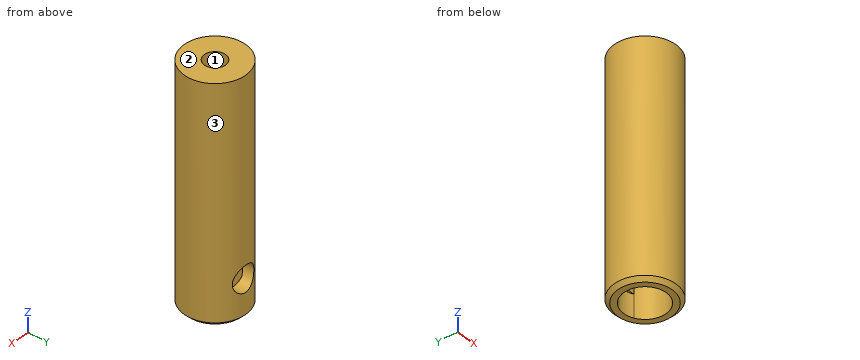
```python
from build123d import *

# Parameters (mm, degrees)
ESQUISSE1_R             = 4.075
BOSS_EXTRU_1_DEPTH      = 30.6
ENL_V_MAT_EXTRU_1_DEPTH = 14
ESQUISSE3_R             = 2.8
ENL_V_MAT_EXTRU_2_DEPTH = 3
CHANFREIN1_SIZE         = 0.5
ESQUISSE5_R             = 1.4
ENL_V_MAT_EXTRU_4_DEPTH = 10
D_GAGEMENT_M31_D        = 3.4
D_GAGEMENT_M31_DEPTH    = 4
D_GAGEMENT_M31_TIP      = 1.021463052


with BuildPart() as part:
    # Esquisse1 → Boss.-Extru.1 (new body)
    with BuildSketch(Plane.XY):
        Circle(ESQUISSE1_R)
    extrude(amount=BOSS_EXTRU_1_DEPTH)

    # Esquisse2 → Enlèv. mat.-Extru.1 (cut)
    with BuildSketch(Plane(origin=(0, 0, 0), x_dir=(-1, 0, 0), z_dir=(0, 0, -1))):
        with BuildLine():
            Line((-1.260952021, 2.5), (1.260952021, 2.5))
            ThreePointArc((1.260952021, 2.5), (0, -2.8), (-1.260952021, 2.5))
        make_face()
    extrude(amount=-ENL_V_MAT_EXTRU_1_DEPTH, mode=Mode.SUBTRACT)

    # Esquisse3 → Enlèv. mat.-Extru.2 (cut)
    with BuildSketch(Plane(origin=(0, 0, 0), x_dir=(-1, 0, 0), z_dir=(0, 0, -1))):
        Circle(ESQUISSE3_R)
    extrude(amount=-ENL_V_MAT_EXTRU_2_DEPTH, mode=Mode.SUBTRACT)

    # Chanfrein1
    chanfrein1_edges = [part.edges().sort_by_distance(p)[0] for p in [
        (-4.075, 0, 0),
    ]]
    chamfer(chanfrein1_edges, length=CHANFREIN1_SIZE)

    # Esquisse5 → Enlèv. mat.-Extru.4 (cut)
    with BuildSketch(Plane.XY.offset(30.6)):
        Circle(ESQUISSE5_R)
    extrude(amount=-ENL_V_MAT_EXTRU_4_DEPTH, mode=Mode.SUBTRACT)

    # Dégagement M31
    with Locations(Plane(origin=(0, 4.075, 0), x_dir=(1, 0, 0), z_dir=(0, 1, 0))):
        with Locations((0, -5)):
            Hole(D_GAGEMENT_M31_D / 2, depth=D_GAGEMENT_M31_DEPTH)
            with Locations((0, 0, -(D_GAGEMENT_M31_DEPTH + D_GAGEMENT_M31_TIP / 2))):  # 118° drill point
                Cone(0, D_GAGEMENT_M31_D / 2, D_GAGEMENT_M31_TIP, mode=Mode.SUBTRACT)


solid = part.part
```
Check sheet for the modelled part. Datum: model origin and axes. Units: mm. Face numbers are marked on the shaded views. Round coordinates to 2 decimals unless told otherwise and drop trailing zeros. Loops run counter-clockwise (first coordinate to the right, second up) from the corner with the lowest first, then second, coordinate; pieces in that order, holes last. Notation, with made-up numbers: (37, 28.5) - (89, 28.5) arc R30 cw to (89, 65.5) - close; hole circle Ø2 at (84.25, 70.5). An arc over 180 degrees is marked (long way). Write item = value, one per line. Start each with the question number.
Q1. Section check A-A (x = 0). Record the boundary of the cut face in (y, z) (3 decimals).
Q2. Depth check by flat-ended pin: P1, Ø1.5, axis at x = -2.5, y = -1.5, coming from the -Z side; P2, Ø2, axis at x = 1.5, z = 7.5, coming from the +Y side; P3, Ø3.5, axis at x = 0, y = 0, coming from the -Z side. Enter the tip coordinate at first touch or a pass-through.
Q3. Thickness scan on L1, parallel to Y at x = 0, z = 25.5 (3 decimals); L2, parallel to Y at x = 0, z = 10.5 (3 decimals); L3, parallel to X at y = 1.75, z = 9.5. Record the ranges inside material, lowest first.
Q4. Section check D-D (z = 29). Record the boundary of the cut face in (x, y) (3 decimals), plus the area to 3 significant figures.
Q5. Section check C-C (z = 13.5). Record the boundary of the cut face in (x, y) (3 decimals).
Q6. Release check for a two-part mould opening along X. For the marked faces 1, 2 and 3 record: pulls with the +X half, pulls with the -X half, needs draft (parallel to the pull), parting line crosses it, or undercut.
Q7. Section check B-B (y = 0). Record the boundary of the cut face in (x, z) (3 decimals), plus the area to 3 significant figures.
Derived:
q1.outline = (-4.075, 0.5) - (-3.575, 0) - (-2.8, 0) - (-2.8, 14) - (2.5, 14) - (2.5, 6.7) - (4.075, 6.7) - (4.075, 30.6) - (1.4, 30.6) - (1.4, 20.6) - (-1.4, 20.6) - (-1.4, 30.6) - (-4.075, 30.6) - close; (2.5, 3) - (2.8, 3) - (2.8, 0) - (3.575, 0) - (4.075, 0.5) - (4.075, 3.3) - (2.5, 3.3) - close
q2.P1 = 0
q2.P2 = 4.04
q2.P3 = 14
q3.L1 = -4.075 to -1.4, 1.4 to 4.075
q3.L2 = -4.075 to -2.8, 2.5 to 4.075
q3.L3 = -3.68 to -2.19, 2.19 to 3.68
q4.outline = circle Ø8.15 at (0, 0); hole circle Ø2.8 at (0, 0)
q4.area = 46.0 mm^2
q5.outline = circle Ø8.15 at (0, 0); hole (-1.261, 2.5) arc R2.8 ccw (long way) to (1.261, 2.5) - close
q6.face_1 = undercut
q6.face_2 = needs draft
q6.face_3 = parting line crosses it
q7.outline = (-4.075, 0.5) - (-3.575, 0) - (-2.8, 0) - (-2.8, 14) - (2.8, 14) - (2.8, 0) - (3.575, 0) - (4.075, 0.5) - (4.075, 30.6) - (1.4, 30.6) - (1.4, 20.6) - (-1.4, 20.6) - (-1.4, 30.6) - (-4.075, 30.6) - close
q7.area = 143 mm^2
